The model under review builds one solid part; all positions refer to its coordinate system, in mm. Face numbers are marked on the shaded views. A direction names the side the tool comes from. Round coordinates to 2 decimals unless told otherwise and drop trailing zeros. Order: outer loops, then holes, each group sorted by start corner. A loop starts at its lowest first (then second) coordinate and runs counter-clockwise, first axis right, second up. Notation, with made-up numbers: (62.25, 39) -> (88.25, 39) arc R22 cw to (88.25, 54) -> close; hole circle Ø5 at (8, 85). An arc over 180 degrees is marked (long way). Return JSON: item names as keys, results as strings. Group by question number.
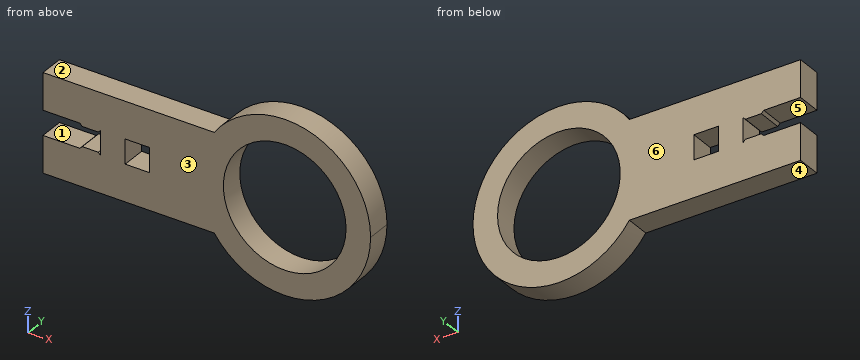
from build123d import *

# Parameters (mm, degrees)
F0_R     = 5
F0_W     = 3
F0_H     = 3
F1_DEPTH = 2


with BuildPart() as f1:
    # F0 (on Front) → F1 (new body)
    with BuildSketch(Plane.XZ):
        with BuildLine():
            ThreePointArc((18.958906, -4), (26.799663, -6.67877), (31.703468, 0))
            ThreePointArc((31.703468, 0), (26.799663, 6.67877), (18.958906, 4))
            ThreePointArc((18.958906, 4), (18.191959, 2.569095), (17.775265, 1))
            ThreePointArc((17.775265, 1), (17.703468, 0), (17.775265, -1))
            ThreePointArc((17.775265, -1), (18.191959, -2.569095), (18.958906, -4))
        make_face()
        with Locations((24.703468, 0)):
            Circle(F0_R, mode=Mode.SUBTRACT)
        with BuildLine():
            ThreePointArc((17.775265, 1), (18.191959, 2.569095), (18.958906, 4))
            Line((18.958906, 4), (8.003468, 4))
            Line((8.003468, 4), (8.003468, 1))
            Line((8.003468, 1), (9.703468, 1))
            Line((9.703468, 1), (11.703468, 1))
            Line((11.703468, 1), (13.703468, 1))
            Line((13.703468, 1), (17.775265, 1))
        make_face()
        with BuildLine():
            ThreePointArc((17.775265, -1), (17.703468, 0), (17.775265, 1))
            Line((17.775265, 1), (13.703468, 1))
            Line((13.703468, 1), (13.703468, -1))
            Line((13.703468, -1), (17.775265, -1))
        make_face()
        Polygon((11.703468, -1), (11.703468, 1), (9.703468, 1), (9.703468, 0), (9.703468, -1), align=None)
        with BuildLine():
            Line((8.003468, -4), (18.958906, -4))
            ThreePointArc((18.958906, -4), (18.191959, -2.569095), (17.775265, -1))
            Line((17.775265, -1), (13.703468, -1))
            Line((13.703468, -1), (11.703468, -1))
            Line((11.703468, -1), (9.703468, -1))
            Line((9.703468, -1), (8.003468, -1))
            Line((8.003468, -1), (8.003468, -4))
        make_face()
        Polygon((8.203468, -0.8), (8.003468, -1), (9.703468, -1), (9.503468, -0.8), align=None)
        Polygon((9.703468, 1), (8.003468, 1), (8.203468, 0.8), (9.503468, 0.8), align=None)
        with Locations((6.503468, 2.5)):
            Rectangle(F0_W, F0_H)
        with Locations((6.503468, -2.5)):
            Rectangle(F0_W, F0_H)
    extrude(amount=F1_DEPTH)


solid = f1.part
Item 1: The part is to be moulded in two halves that separate along Z. For the marked faces 1, 2, 3 and 4, say which applies: +Z half, -Z half, draft (parallel to the pull), parting line (faces both ways), or undercut.
Item 2: Consider section C-C on x = 26.25. State the section outline as (y, z) points, plus the area to 3 significant figures.
Item 3: Consider section D-D on z = 6. State the section outline as (x, y) points, plus the area to 3 significant figures.
Item 4: Consider section B-B on z = -3.75. State the section outline as (x, y) points, plus the area to 3 significant figures.
Item 5: For the marked faces 5 and 6, list the 3-axis set-ups (+Z, -Z, +X, -X, +Y, -Y) from which the entire face can be reached by the end or side of a thin tool; tool diameter is ignored.
Item 6: Consider section A-A on y = -1.6. State the section outline as (x, z) points.
Item 7: Wall thickness on line 1 along Z through (x, y) = (24.5, -1.35); line 2 along Z through (x, y) = (9.5, -0.9); line 3 along Z through (x, y) = (15.75, -0.05): over which ranges is each line inside the solid? List them lowest first.
Item 8: Insertion check: pin 1 Ø1 at (x, y) = (9, -0.5) entering from +Z; pin 2 Ø0.6 at (x, y) = (9, -1) entering from -Z. Each pin has a flat end and moves straight along its axis. Give the tip position at first contact, or say it passes through.
Values:
{
 "1": {"face 1": "undercut", "face 2": "+Z half", "face 3": "draft", "face 4": "-Z half"},
 "2": {"outline": "(-2, -6.83) -> (0, -6.83) -> (0, -4.75) -> (-2, -4.75) -> close; (-2, 4.75) -> (0, 4.75) -> (0, 6.83) -> (-2, 6.83) -> close", "area": "8.29 mm^2"},
 "3": {"outline": "(21.1, -2) -> (28.31, -2) -> (28.31, 0) -> (21.1, 0) -> close", "area": "14.4 mm^2"},
 "4": {"outline": "(5, -2) -> (21.4, -2) -> (21.4, 0) -> (5, 0) -> close; (28.01, -2) -> (30.61, -2) -> (30.61, 0) -> (28.01, 0) -> close", "area": "38.0 mm^2"},
 "5": {"face 5": "-X, +Y, -Y", "face 6": "+Z, -Z, +X, -X, +Y"},
 "6": {"outline": "(5, -4) -> (18.96, -4) arc R7 ccw (long way) to (18.96, 4) -> (5, 4) -> (5, 1) -> (8, 1) -> (8.2, 0.8) -> (9.5, 0.8) -> (9.7, 1) -> (9.7, -1) -> (9.5, -0.8) -> (8.2, -0.8) -> (8, -1) -> (5, -1) -> close; hole (11.7, -1) -> (13.7, -1) -> (13.7, 1) -> (11.7, 1) -> close; hole circle Ø10 at (24.7, 0)"},
 "7": {"line 1": "-7 to -5, 5 to 7", "line 2": "-4 to -0.8, 0.8 to 4", "line 3": "-4 to 4"},
 "8": {"pin 1": "z = 4", "pin 2": "z = -4"}
}
